Answer from the drawing. Dimensions are ordinates in mm from the lowest x, y and z of the part. Round coordinates to 2 decimals unless told otherwise and drop trailing zeros. Write each loop counter-clockwise with the first axis right and the second up, starting at its lowest first coordinate (ties: lowest second). Pieces come first, ordered by that corner, then holes. Notation, with made-up numbers: (4.5, 50.5) - (35.5, 50.5) arc R17 ccw to (35.5, 81.5) - close; hole circle Ø10 at (44, -34.75). An arc over 180 degrees is marked (long way). Return JSON: item names as keys, results as strings. Group by question number.
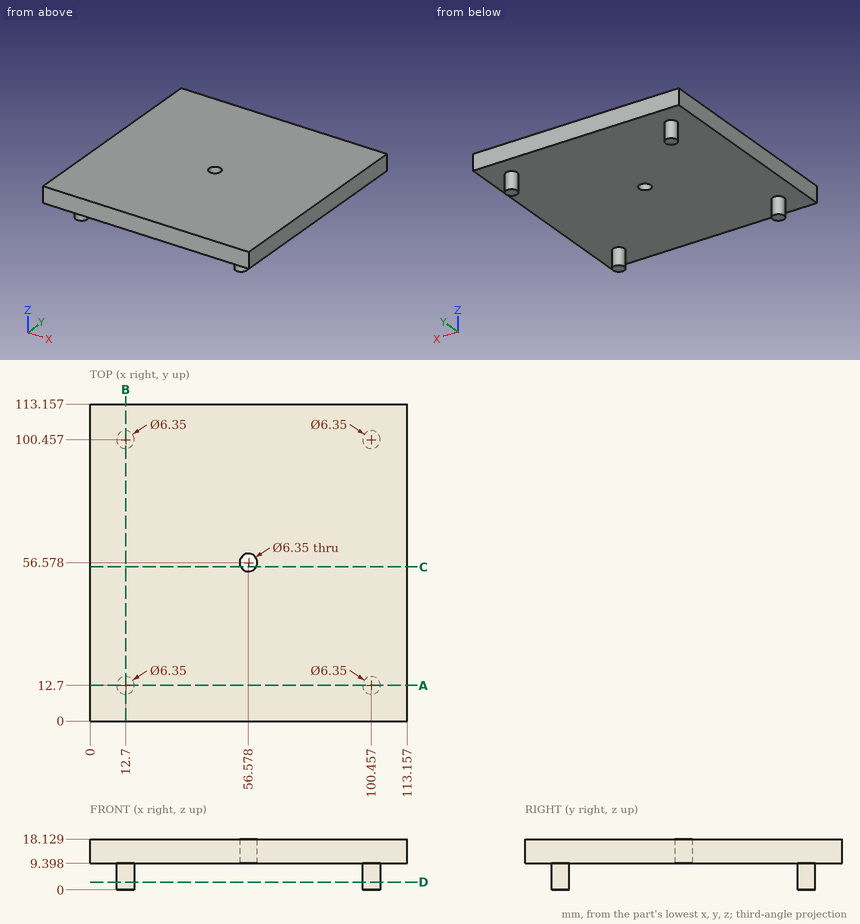
(1) Find section A-A (y = 12.7). Write down the section's boundary in (x, z) (1 decimal), plus the area to 3 significant figures.
(2) Find section D-D (z = 2.75). State how many separate pieces and enclosed holes the cut face has, plus the area to 3 significant figures.
(3) Find section C-C (y = 55). Write down the section's boundary in (x, z).
(4) A flat-ended cylindrical pin translates along its axis: pin 1 (1 mm diameter, centred on x = 38, y = 25.5, fed in from -Z). Find the tip coordinate at first contact, or state that the pin passes through.
(5) Consider line 1 (Z direction, x = 72, y = 44); line 2 (X direction, y = 15, z = 8.5) (1 decimal); line 3 (Y direction, x = 54.5, z = 16.5) (1 decimal). Determine where each line is inside the solid, lowest interval first.
Check sheet entries:
{
 "1": {"outline": "(0, 9.4) - (9.5, 9.4) - (9.5, 0) - (15.9, 0) - (15.9, 9.4) - (97.3, 9.4) - (97.3, 0) - (103.6, 0) - (103.6, 9.4) - (113.2, 9.4) - (113.2, 18.1) - (0, 18.1) - close", "area": "1,110 mm^2"},
 "2": {"separate pieces": "4", "enclosed holes": "0", "area": "127 mm^2"},
 "3": {"outline": "(0, 9.4) - (53.82, 9.4) - (53.82, 18.13) - (0, 18.13) - close; (59.33, 9.4) - (113.16, 9.4) - (113.16, 18.13) - (59.33, 18.13) - close"},
 "4": {"pin 1": "stops at z = 9.4"},
 "5": {"line 1": "z = 9.4 to 18.13", "line 2": "x = 10.5 to 14.9, 98.3 to 102.6", "line 3": "y = 0 to 54.2, 59 to 113.2"}
}
